The listing builds one solid part. Answer for the finished solid, in the listing's coordinates (mm). Face numbers are marked on the shaded views. A direction names the side the tool comes from. Round coordinates to 2 decimals unless told otherwise and drop trailing zeros. Order: outer loops, then holes, each group sorted by start corner. A loop starts at its lowest first (then second) coordinate and runs counter-clockwise, first axis right, second up. Notation, with made-up numbers: (69, 59) -> (124, 59) arc R31 ccw to (124, 91) -> close; hole circle Ø6 at (-24, 41.5). An arc over 180 degrees is marked (long way). Answer in a Markdown table with one row per item. Add a question column.
```python
from build123d import *

# Parameters (mm, degrees)
SKETCH1_R                           = 2.38125
BOSS_EXTRUDE1_DEPTH                 = 3.175
F_9_64_0_14063_DIAMETER_HOLE1_D     = 3.572002
F_9_64_0_14063_DIAMETER_HOLE1_DEPTH = 3.175
FILLET1_R                           = 2.54
SKETCH9_W                           = 28.956
SKETCH9_H                           = 9.242923456
SKETCH9_R                           = 1.397
SKETCH9_H_2                         = 9.1095327
BOSS_EXTRUDE3_DEPTH                 = 16.51
SKETCH10_R                          = 3.429
CUT_EXTRUDE1_DEPTH                  = 6.35
SKETCH11_W                          = 8.636
SKETCH11_H                          = 9.242923456
CUT_EXTRUDE2_DEPTH                  = 7.62


with BuildPart() as part:
    # Sketch1 → Boss-Extrude1 (new body)
    with BuildSketch(Plane(origin=(0, 0, 0), x_dir=(1, 0, 0), z_dir=(0, 1, 0))):
        Polygon((18.288, -9.6647), (22.225, -9.6647), (22.225, -17.3228), (18.288, -17.3228), (18.288, -23.8125), (-18.288, -23.8125), (-18.288, -17.3228), (-22.225, -17.3228), (-22.225, -9.6647), (-18.288, -9.6647), (-18.288, 9.6647), (-22.225, 9.6647), (-22.225, 17.3228), (-18.288, 17.3228), (-18.288, 55.5625), (18.288, 55.5625), (18.288, 17.3228), (22.225, 17.3228), (22.225, 9.6647), (18.288, 9.6647), align=None)
        with Locations((0, 0.004315819)):
            Circle(SKETCH1_R, mode=Mode.SUBTRACT)
    extrude(amount=BOSS_EXTRUDE1_DEPTH)

    # 9/64 (0.14063) Diameter Hole1
    with Locations(Plane.XZ):
        with Locations((18.287999999, -13.474700001), (18.288, 13.466068362), (-18.288, -13.470384182), (-18.288, 13.470384182)):
            Hole(F_9_64_0_14063_DIAMETER_HOLE1_D / 2, depth=F_9_64_0_14063_DIAMETER_HOLE1_DEPTH)

    # Fillet1
    fillet1_edges = [part.edges().sort_by_distance(p)[0] for p in [
        (18.288, 1.5875, 23.8125),
        (-18.288, 1.5875, 23.8125),
        (-18.288, 1.5875, 17.3228),
        (-18.288, 1.5875, 9.6647),
        (-18.288, 1.5875, -9.6647),
        (-18.288, 1.5875, -17.3228),
        (-18.288, 1.5875, -55.5625),
        (18.288, 1.5875, -55.5625),
        (18.288, 1.5875, -17.3228),
        (18.288, 1.5875, -9.6647),
        (18.288, 1.5875, 9.6647),
        (18.288, 1.5875, 17.3228),
    ]]
    fillet(fillet1_edges, radius=FILLET1_R)

    # Sketch9 → Boss-Extrude3 (add)
    with BuildSketch(Plane(origin=(0, 0, 0), x_dir=(1, 0, 0), z_dir=(0, 1, 0))):
        with Locations((0, -19.191038272)):
            Rectangle(SKETCH9_W, SKETCH9_H)
        with Locations((-7.9375, -18.25625)):
            Circle(SKETCH9_R, mode=Mode.SUBTRACT)
        with Locations((7.9375, -18.25625)):
            Circle(SKETCH9_R, mode=Mode.SUBTRACT)
        with Locations((0.012736117, 51.00773365)):
            Rectangle(SKETCH9_W, SKETCH9_H_2)
        with Locations((-7.9375, 49.76495)):
            Circle(SKETCH9_R, mode=Mode.SUBTRACT)
        with Locations((7.9375, 49.76495)):
            Circle(SKETCH9_R, mode=Mode.SUBTRACT)
    extrude(amount=BOSS_EXTRUDE3_DEPTH)

    # Sketch10 → Cut-Extrude1 (cut)
    with BuildSketch(Plane.XZ):
        with Locations((7.9375, 18.25625)):
            Circle(SKETCH10_R)
        with Locations((-7.9375, 18.25625)):
            Circle(SKETCH10_R)
        with Locations((7.9375, -49.76495)):
            Circle(SKETCH10_R)
        with Locations((-7.9375, -49.76495)):
            Circle(SKETCH10_R)
    extrude(amount=-CUT_EXTRUDE1_DEPTH, mode=Mode.SUBTRACT)

    # Sketch11 → Cut-Extrude2 (cut)
    with BuildSketch(Plane(origin=(0, 16.51, 0), x_dir=(1, 0, 0), z_dir=(0, 1, 0))):
        with Locations((0, -19.191038272)):
            Rectangle(SKETCH11_W, SKETCH11_H)
    extrude(amount=-CUT_EXTRUDE2_DEPTH, mode=Mode.SUBTRACT)


solid = part.part
```
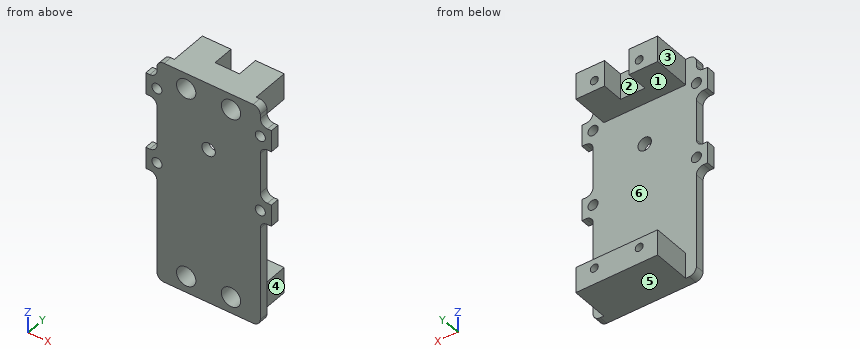
1. The part is cut by section B-B (y = 13.5). Give the vertices of the cut face in (x, z).
2. The part is cut by section D-D (x = -17.5). Give the vertices of the cut face in (y, z) (3 decimals), then the cut area to 3 significant figures.
3. The part is cut by section C-C (y = 7.5). Give the vertices of the cut face in (x, z), then the cut area to 3 significant figures.
4. Each of these flat-tipped pins is pushed along its axis until it touches: pin 1 (1.1 mm diameter, centred on x = 21.5, y = 1, fed in from -Z); pin 2 (2 mm diameter, centred on x = 9, z = 19, fed in from -Y); pin 3 (0.7 mm diameter, centred on y = 1.5, z = 20.5, fed in from +X). Where does it stop, or does it pass through?
5. For the marked faces 1, 2 and 3, determine the directions among +Z, -Z, +X, -X, +Y, -Y from which every point of the face is accessible in a straight line to the end or side of a thin tool.
6. The part is cut by section A-A (x = 0). Give the vertices of the cut face in (y, z) (1 decimal).
7. The mould has two halves that part along Z. Classify the marked faces 4, 5 and 6: released by +Z, released by -Z, zero draft, split by the parting line, or undercut.
8. Straight lines are drawn through the part: line 1 along Z through (x, y) = (13, 12.75); line 2 along X through (y, z) = (15, 18.5); line 3 along Z through (x, y) = (-7.5, 4). For each, find the intervals that lie inside material, in ascending order.
Report:
| question | item | result |
|---|---|---|
| 1 | outline | (-14.48, 14.57) -> (-4.32, 14.57) -> (-4.32, 23.81) -> (-14.48, 23.81) -> close; (-14.47, -55.56) -> (14.49, -55.56) -> (14.49, -46.45) -> (-14.47, -46.45) -> close; (4.32, 14.57) -> (14.48, 14.57) -> (14.48, 23.81) -> (4.32, 23.81) -> close; hole circle Ø2.79 at (-7.94, -49.76); hole circle Ø2.79 at (-7.94, 18.26); hole circle Ø2.79 at (7.94, -49.76); hole circle Ø2.79 at (7.94, 18.26) |
| 2 | outline | (0, -54.862) -> (3.175, -54.862) -> (3.175, -15.073) -> (0, -15.073) -> close; (0, -11.868) -> (3.175, -11.868) -> (3.175, 11.868) -> (0, 11.868) -> close; (0, 15.073) -> (3.175, 15.073) -> (3.175, 23.112) -> (0, 23.112) -> close |
| 2 | area | 227 mm^2 |
| 3 | outline | (-14.48, 14.57) -> (14.48, 14.57) -> (14.48, 23.81) -> (-14.48, 23.81) -> close; (-14.47, -55.56) -> (14.49, -55.56) -> (14.49, -46.45) -> (-14.47, -46.45) -> close; hole circle Ø2.79 at (-7.94, -49.76); hole circle Ø2.79 at (-7.94, 18.26); hole circle Ø2.79 at (7.94, -49.76); hole circle Ø2.79 at (7.94, 18.26) |
| 3 | area | 507 mm^2 |
| 4 | pin 1 | stops at z = -17.32 |
| 4 | pin 2 | stops at y = 6.35 |
| 4 | pin 3 | stops at x = 18.29 |
| 5 | face 1 | +X, -X, +Y |
| 5 | face 2 | +Z, +Y |
| 5 | face 3 | +Z, -Z, -X, +Y |
| 6 | outline | (0, -55.6) -> (16.5, -55.6) -> (16.5, -46.5) -> (3.2, -46.5) -> (3.2, -2.4) -> (0, -2.4) -> close; (0, 2.4) -> (3.2, 2.4) -> (3.2, 14.6) -> (8.9, 14.6) -> (8.9, 23.8) -> (0, 23.8) -> close |
| 7 | face 4 | zero draft |
| 7 | face 5 | released by -Z |
| 7 | face 6 | undercut |
| 8 | line 1 | z = -55.56 to -46.45, 14.57 to 23.81 |
| 8 | line 2 | x = -14.48 to -9.31, -6.56 to -4.32, 4.32 to 6.56, 9.31 to 14.48 |
| 8 | line 3 | z = -55.56 to -53.17, 14.57 to 14.86, 21.66 to 23.81 |
